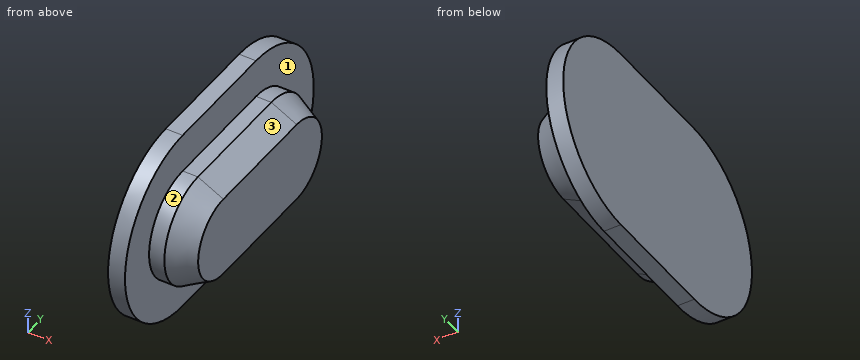
from build123d import *

# Parameters (mm, degrees)
EXTRUDE008_DEPTH = 1
EXTRUDE007_DEPTH = 2.4
CHAMFER004_SIZE2 = 0.8
CHAMFER004_SIZE  = 1.5


with BuildPart() as extrude008:
    # Sketch009 (on Sketch) → Extrude008 (new body)
    with BuildSketch(Plane(origin=(-47.25, 0, 0), x_dir=(0, -1, 0), z_dir=(-1, 0, 0))):
        with BuildLine():
            ThreePointArc((0.75, 12.5), (-4.75, 7), (0.75, 1.5))
            Line((0.75, 1.5), (7.75, 1.5))
            ThreePointArc((7.75, 1.5), (13.25, 7), (7.75, 12.5))
            Line((7.75, 12.5), (0.75, 12.5))
        make_face()
    extrude(amount=EXTRUDE008_DEPTH)


with BuildPart() as deckel_usb:
    # Sketch008 (on Sketch) → Extrude007 (new body)
    with BuildSketch(Plane(origin=(-47.25, 0, 0), x_dir=(0, -1, 0), z_dir=(-1, 0, 0))):
        with BuildLine():
            ThreePointArc((0.75, 10.2), (-2.45, 7), (0.75, 3.8))
            Line((0.75, 3.8), (7.75, 3.8))
            ThreePointArc((7.75, 3.8), (10.95, 7), (7.75, 10.2))
            Line((7.75, 10.2), (0.75, 10.2))
        make_face()
    extrude(amount=-EXTRUDE007_DEPTH)

    # Chamfer004
    chamfer004_edges = [deckel_usb.edges().sort_by_distance(p)[0] for p in [
        (-44.85, -4.25, 3.8),
    ]]
    chamfer004_side = deckel_usb.faces().sort_by_distance((-46.05, -4.25, 3.8))[0]
    chamfer(chamfer004_edges, length=CHAMFER004_SIZE, length2=CHAMFER004_SIZE2, reference=chamfer004_side)

    # Connect001: union Extrude008
    add(extrude008.part)


solid = deckel_usb.part
Design review of the part built by this model. Coordinates are the model's own, in mm. Face numbers are marked on the shaded views. A direction names the side the tool comes from. Give positions to 0.01 mm unless a question says otherwise; leave off trailing zeros. Loops run counter-clockwise (first coordinate to the right, second up) from the corner with the lowest first, then second, coordinate; pieces in that order, holes last. Notation, with made-up numbers: M 9.25,53.25 L 18.25,53.25 A27 ccw 18.25,69.25 Z; hole C 67.5,55.5 d9. An arc over 180 degrees is marked long. Write item = value, one per line.
Q1. We need section C-C (x = -47.9). Give the boundary of the cut face in (y, z).
Output values:
outline = M -7.75,1.5 L -0.75,1.5 A5.5 ccw -0.75,12.5 L -7.75,12.5 A5.5 ccw Z
Q2. We need section D-D (x = -46.65). Give the boundary of the cut face in (y, z), plus the area to 3 significant figures.
Output values:
outline = M -7.75,3.8 L -0.75,3.8 A3.2 ccw -0.75,10.2 L -7.75,10.2 A3.2 ccw Z
area = 77.0 mm^2
Q3. To check wall thickness, follow line 1 (X direction, y = 3.5, z = 4.5); line 2 (Z direction, x = -46.8, y = -5.25); line 3 (Y direction, x = -47.15, z = 7). State the ranges of each line that lie inside material, in increasing order. Write a range as [from, to].
Output values:
line_1 = [-48.25, -47.25]
line_2 = [3.8, 10.2]
line_3 = [-10.95, 2.45]
Q4. For the marked faces 1, 2 and 3, list the 3-axis set-ups (+Z, -Z, +X, -X, +Y, -Y) from which the entire face can be reached by the end or side of a thin tool; tool diameter is ignored.
Output values:
face_1 = +X
face_2 = +X, -Y
face_3 = +Z, +X, +Y, -Y
Q5. Insertion check: pin 1 (1 mm diameter, centred on x = -45.5, z = 3.5, fed in from +Y); pin 2 (1 mm diameter, centred on x = -46.5, y = -4.5, fed in from -Z). Each pin has a flat end and moves straight along its axis. Give the tip position at first contact, or say it passes through.
Output values:
pin_1 = through
pin_2 = 3.8
Q6. We need section B-B (y = -2.25). Give the boundary of the cut face in (x, z).
Output values:
outline = M -48.25,1.5 L -47.25,1.5 L -47.25,3.8 L -46.35,3.8 L -44.85,4.6 L -44.85,9.4 L -46.35,10.2 L -47.25,10.2 L -47.25,12.5 L -48.25,12.5 Z
Q7. We need section A-A (z = 7). Give the boundary of the cut face in (x, y), plus the area to 3 significant figures.
Output values:
outline = M -48.25,-13.25 L -47.25,-13.25 L -47.25,-10.95 L -46.35,-10.95 L -44.85,-10.15 L -44.85,1.65 L -46.35,2.45 L -47.25,2.45 L -47.25,4.75 L -48.25,4.75 Z
area = 49.0 mm^2
